Here's the drawing with two shaded views (mm, measured from the low corner). I have some questions. A direction names the side the tool comes from. Coordinates: 2 decimals unless noted, no trailing zeros. Loops run counter-clockwise (first coordinate to the right, second up) from the corner with the lowest first, then second, coordinate; pieces in that order, holes last. Notation, with made-up numbers: M 11.25,78.25 L 60.25,78.25 A31 cw 60.25,117.25 Z; hole C 45.5,39.25 d9. An arc over 180 degrees is marked long. Return JSON: item names as keys, results as strings. Group by question number.
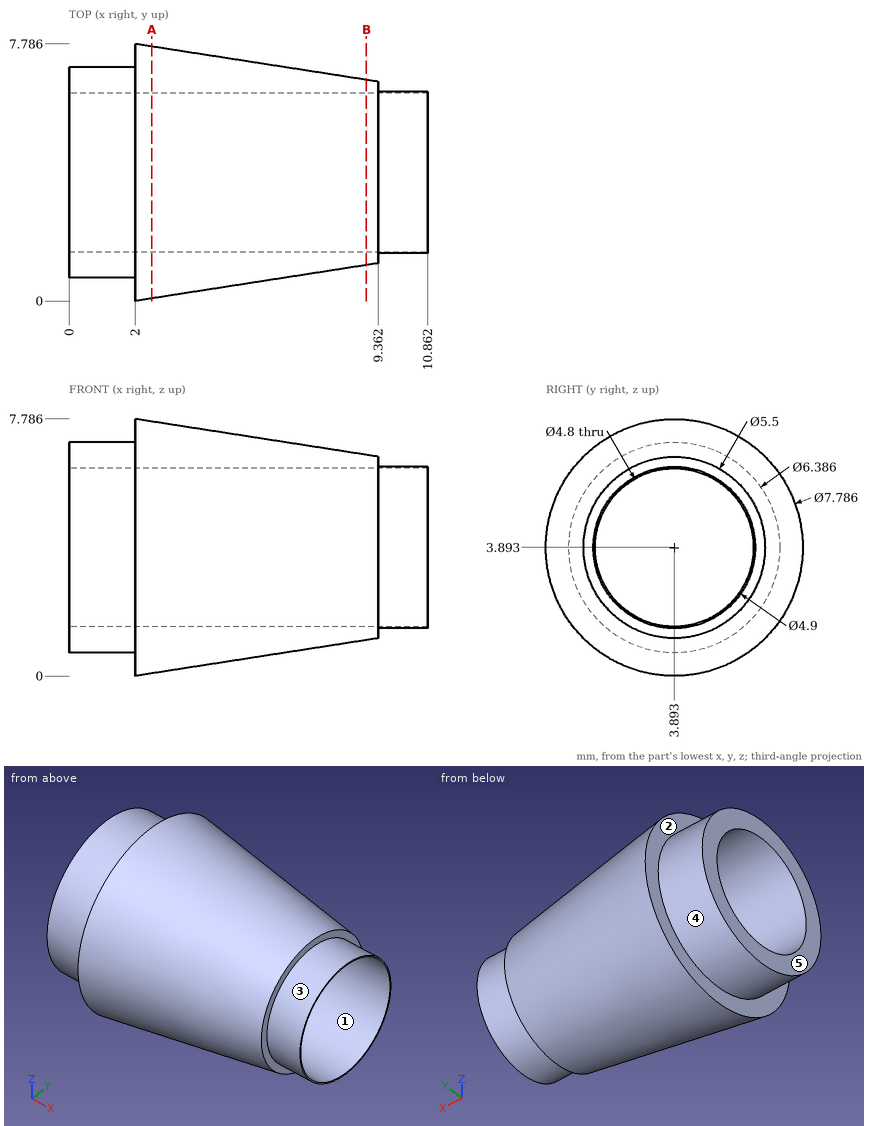
1) If we mould it in two halves opening along Z, with no side actions, what happens to the marked faces 1, 2 and 3? For each: +Z half, -Z half, draft (parallel to the pull), parting line (faces both ways), or undercut.
2) If I drill on line 1 (X direction, y = 1.25, z = 4); line 2 (Z direction, x = 6, y = 5.5) (1 decimal); line 3 (Z direction, x = 1, y = 2) (1 decimal), over which ranges is the centre line in solid material (lowest first)? Write a range as from..to.
3) For the marked faces 4 and 5, which set-ups out of +Z, -Z, +X, -X, +Y, -Y let a thin tool reach every point of the face, with its end or its side?
4) Suppose I cut it at A-A, the plane x = 2.5. List the corners of the cut face in (y, z) for me (1 decimal), then the cut area to 3 significant figures.
5) For pin 1 (4 mm diameter, centred on x = 8, z = 3.5, fed in from +Y); pin 2 (4 mm diameter, centred on x = 4.5, y = 5.5, fed in from -Z); pin 3 (4 mm diameter, centred on x = 5.5, z = 6.5, fed in from +Y), each with a flat end and sliding along its axis, tell me the tip position at first contact or that it passes through.
6) Suppose I cut it at B-B, the plane x = 9. List the corners of the cut face in (y, z) for me.
Returned:
{
 "1": {"face 1": "undercut", "face 2": "draft", "face 3": "parting line"},
 "2": {"line 1": "x = 0..9.36", "line 2": "z = 1..2.1, 5.7..6.7", "line 3": "z = 1.3..2.4, 5.4..6.5"},
 "3": {"face 4": "-X", "face 5": "+Z, -Z, -X, +Y, -Y"},
 "4": {"outline": "C 3.9,3.9 d7.6; hole C 3.9,3.9 d4.8", "area": "27.6 mm²"},
 "5": {"pin 1": "stops at y = 7.16", "pin 2": "stops at z = 0.16", "pin 3": "stops at y = 7.29"},
 "6": {"outline": "C 3.89,3.89 d5.61; hole C 3.89,3.89 d4.8"}
}
